The listing builds one solid part. Answer for the finished solid, in the listing's coordinates (mm). Face numbers are marked on the shaded views. Give positions to 0.01 mm unless a question says otherwise; leave off trailing zeros. Write each loop counter-clockwise with the first axis right and the second up, starting at its lowest first coordinate (ties: lowest second). Pieces come first, ordered by that corner, then holes. Notation, with made-up numbers: M 47.25,72.5 L 71.25,72.5 A27 cw 71.25,110.5 Z; hole C 51.5,-28.75 d11. An arc over 180 degrees is marked long. Return JSON: item names as keys, results as strings.
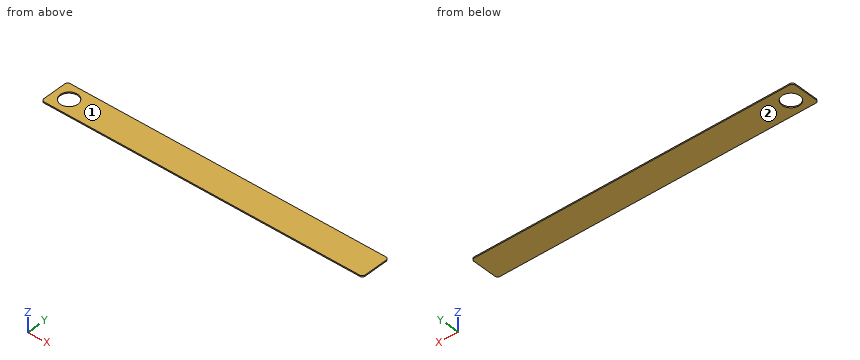
from build123d import *

# Parameters (mm, degrees)
SKETCH1_R           = 1.5
BOSS_EXTRUDE1_DEPTH = 0.2
SCALE6_SCALE        = 0.7


with BuildPart() as part:
    # Sketch1 → Boss-Extrude1 (new body)
    with BuildSketch(Plane.XY):
        with BuildLine():
            Line((-26.75, 2.5), (26.75, 2.5))
            ThreePointArc((26.75, 2.5), (27.103553391, 2.353553391), (27.25, 2))
            Line((27.25, 2), (27.25, -2))
            ThreePointArc((27.25, -2), (27.103553391, -2.353553391), (26.75, -2.5))
            Line((26.75, -2.5), (-26.75, -2.5))
            ThreePointArc((-26.75, -2.5), (-27.103553391, -2.353553391), (-27.25, -2))
            Line((-27.25, -2), (-27.25, 2))
            ThreePointArc((-27.25, 2), (-27.103553391, 2.353553391), (-26.75, 2.5))
        make_face()
        with Locations((-24.75, 0)):
            Circle(SKETCH1_R, mode=Mode.SUBTRACT)
    extrude(amount=BOSS_EXTRUDE1_DEPTH)


with BuildPart() as part_1:
    # Scale6: scaled about (0.659639326, 0, 0.1)
    add(part.part.scale(SCALE6_SCALE).moved(Location((0.197891798, 0, 0.03))))


solid = part_1.part
Item 1: Determine the mould class of the marked faces 1 and 2 for opening direction Z: +Z half, -Z half, draft (parallel to the pull), parting line (faces both ways), or undercut.
Geometry results:
{"face 1": "+Z half", "face 2": "-Z half"}
Item 2: A cutting plane is placed at A-A, the plane z = 0.1. Write down the section's boundary in (x, y).
Geometry results:
{"outline": "M -18.88,-1.4 A0.35 ccw -18.53,-1.75 L 18.92,-1.75 A0.35 ccw 19.27,-1.4 L 19.27,1.4 A0.35 ccw 18.92,1.75 L -18.53,1.75 A0.35 ccw -18.88,1.4 Z; hole C -17.13,0 d2.1"}
Item 3: Find the intervals of material crossed by line 1 (X direction, y = -0.9, z = 0.1); line 2 (X direction, y = -1.55, z = 0.1), in increasing order.
Geometry results:
{"line 1": "x = -18.88 to -17.67, -16.59 to 19.27", "line 2": "x = -18.84 to 19.24"}
Item 4: A cutting plane is placed at B-B, the plane y = 0. Write down the section's boundary in (x, z).
Geometry results:
{"outline": "M -18.88,0.03 L -18.18,0.03 L -18.18,0.17 L -18.88,0.17 Z; M -16.08,0.03 L 19.27,0.03 L 19.27,0.17 L -16.08,0.17 Z"}
